Autodesk Inventor part; units mm, degrees
ref_plane "YZ Plane" through (0, 0, 0) normal (1, 0, 0) x (0, 1, 0)
ref_plane "XZ Plane" through (0, 0, 0) normal (0, 1, 0) x (-1, 0, 0)
ref_plane "XY Plane" through (0, 0, 0) normal (0, 0, 1) x (1, 0, 0)
sketch "スケッチ1" plane through (0, 0, 0) normal (0, 0, 1) x (1, 0, 0)
  circle A0 centre (0, 0) radius 18.13
  dimension "d0" = 36.26
extrude "押し出し1" add sketch "スケッチ1" along normal blind 40
sketch "スケッチ2" plane through (0, 0, 40) normal (0, 0, 1) x (1, 0, 0)
  circle A0 centre (0, 0) radius 19.88
  dimension "d3" = 39.76
extrude "押し出し2" add sketch "スケッチ2" along normal blind 3
sketch "スケッチ3" plane through (0, 0, 0) normal (0, 0, -1) x (-1, 0, 0)
  circle A0 centre (0, 0) radius 19.88
  dimension "d6" = 39.76
extrude "押し出し3" add sketch "スケッチ3" along normal blind 3
sketch "スケッチ4" plane through (0, 0, -3) normal (0, 0, -1) x (-1, 0, 0)
  circle A0 centre (0, 0) radius 2.5
  dimension "d9" = 5
hole "穴1" at (0, 0, -3) direction (0, 0, 1) diameter 5 depth 46
equation "\"BendRadius\" = Thickness"
equation "\"BendReliefWidth\" = Thickness"
equation "\"BendReliefDepth\" = 0.5 * Thickness"
equation "\"CornerReliefSize\" = 4 * Thickness"
equation "\"MinimumRemnant\" = 2 * Thickness"
equation "\"TransitionRadius\" = BendRadius"
equation "\"JacobiRadiusSize\" = BendRadius"
equation "\"GapSize\" = Thickness"
properties part number "nhk13" material "ABS プラスチック"
Source: CAD feature listing. Evaluate the final solid. Frame: model axes, mm. A direction names the side the tool comes from. Round coordinates to 2 decimals unless told otherwise and drop trailing zeros. Loops run counter-clockwise (first coordinate to the right, second up) from the corner with the lowest first, then second, coordinate; pieces in that order, holes last. Notation, with made-up numbers: M -36,38 L -26,38 A20 cw -26,50 Z; hole C -33,37.5 d2. An arc over 180 degrees is marked long. Return JSON: item names as keys, results as strings. Group by question number.
1. Material intervals for line 1 along Y through (x, z) = (0, 26.5); line 2 along Z through (x, y) = (12.5, 15); line 3 along X through (y, z) = (-16.5, 26), sorted ascending. Write a range as from..to.
2. Section query D-D on x = 11.5. Output: boundary loops of the cut face in (y, z).
3. Mould query, pull axis Z, two halves, no side actions, for faces 1 (the face through (10.69, -16.76, 41.48)), 2 (the face through (4, 0, 43)), 3 (the face through (-5, -18, 40)), 4 (the face through (5, -18, 0)). Classes: released by +Z, released by -Z, zero draft, split by the parting line, or undercut.
4. Pin query (flat end, axial travel): pin 1 (10 mm diameter, centred on x = 6.5, z = 2.5, fed in from +Y); pin 2 (1 mm diameter, centred on y = 11, z = 8.5, fed in from -X); pin 3 (1 mm diameter, centred on y = -2, z = 16.5, fed in from -X); pin 4 (6 mm diameter, centred on x = 0, y = 0, fed in from -Z). Return the tip coordinate at first contact, or that it passes through.
5. Section query C-C on y = -5. Output: boundary loops of the cut face in (x, z), and give its area (3 significant figures).
6. Reachability of faces 5 (the face through (-3.93, 17.7, 19.72)), 6 (the face through (2.44, -0.54, 20.32)) from +Z, -Z, +X, -X, +Y, -Y: full face, straight path, thin tool, end or side. Return the list, or none.
7. Section query A-A on y = 0. Output: boundary loops of the cut face in (x, z), and give its area (3 significant figures).
Checks:
{
 "1": {"line 1": "y = -18.13..-2.5, 2.5..18.13", "line 2": "z = -3..0, 40..43", "line 3": "x = -7.51..7.51"},
 "2": {"outline": "M -16.22,-3 L 16.22,-3 L 16.22,0 L 14.02,0 L 14.02,40 L 16.22,40 L 16.22,43 L -16.22,43 L -16.22,40 L -14.02,40 L -14.02,0 L -16.22,0 Z"},
 "3": {"face 1": "zero draft", "face 2": "released by +Z", "face 3": "undercut", "face 4": "undercut"},
 "4": {"pin 1": "stops at y = 19.76", "pin 2": "stops at x = -14.78", "pin 3": "stops at x = -18.07", "pin 4": "stops at z = -3"},
 "5": {"outline": "M -19.24,-3 L 19.24,-3 L 19.24,0 L 17.43,0 L 17.43,40 L 19.24,40 L 19.24,43 L -19.24,43 L -19.24,40 L -17.43,40 L -17.43,0 L -19.24,0 Z", "area": "1,630 mm²"},
 "6": {"face 5": "none", "face 6": "+Z, -Z"},
 "7": {"outline": "M -19.88,-3 L -2.5,-3 L -2.5,43 L -19.88,43 L -19.88,40 L -18.13,40 L -18.13,0 L -19.88,0 Z; M 2.5,-3 L 19.88,-3 L 19.88,0 L 18.13,0 L 18.13,40 L 19.88,40 L 19.88,43 L 2.5,43 Z", "area": "1,460 mm²"}
}
